Source: CAD feature listing. Evaluate the final solid. Frame: model axes, mm. A direction names the side the tool comes from. Give positions to 0.01 mm unless a question says otherwise; leave off trailing zeros. Order: outer loops, then holes, each group sorted by start corner. A loop starts at its lowest first (then second) coordinate and runs counter-clockwise, first axis right, second up.
from build123d import *

# Parameters (mm, degrees)
F0_R      = 3.91
F1_DEPTH  = 25
F1_FACE_R = 3.91
F2_DEPTH  = 2
F3_SIZE   = 1


with BuildPart() as f1:
    # F0 (on Top) → F1 (new body)
    with BuildSketch(Plane.XY):
        Circle(F0_R)
    extrude(amount=-F1_DEPTH)

    # F0 (on Top) + F1_face (on face) → F2 (join)
    with BuildSketch(Plane.XY):
        Polygon((5.284141717, -4.9639043418), (6.9409381205, 2.0942487932), (1.6567964035, 7.058153135), (-5.284141717, 4.9639043418), (-6.9409381205, -2.0942487932), (-1.6567964035, -7.058153135), align=None)
        Circle(F0_R, mode=Mode.SUBTRACT)
    with BuildSketch(Plane.XY):
        Circle(F1_FACE_R)
    extrude(amount=F2_DEPTH)

    # F3
    f3_edges = [f1.edges().sort_by_distance(p)[0] for p in [
        (-3.91, 0, -25),
    ]]
    chamfer(f3_edges, length=F3_SIZE)


solid = f1.part
1) Section query C-C on x = 0. Output: boundary loops of the cut face in (y, z), and give its area (3 significant figures).
Checks:
outline: (-6.56, 0) - (-3.91, 0) - (-3.91, -24) - (-2.91, -25) - (2.91, -25) - (3.91, -24) - (3.91, 0) - (6.56, 0) - (6.56, 2) - (-6.56, 2) - close
area: 221 mm2
2) Section query D-D on y = -4.25. Output: boundary loops of the cut face in (x, z).
Checks:
outline: (-4.65, 0) - (5.45, 0) - (5.45, 2) - (-4.65, 2) - close
3) Ray query, L1, parallel to Z at x = 1.75, y = -5.5; L2, parallel to Y at x = 0, z = -15.5; L3, parallel to Z at x = 3, y = 1.25. Return the intervals inside material, ascending.
Checks:
L1: z = 0 to 2
L2: y = -3.91 to 3.91
L3: z = -24.66 to 2
4) Reachability of faces 1 (the face through (-1.765, 6.026, 0.986)), 2 (the face through (3, -3, 0)) from +Z, -Z, +X, -X, +Y, -Y: full face, straight path, thin tool, end or side. Return the list, or none.
Checks:
face 1: +Z, -Z, -X, +Y
face 2: -Z
5) Section query A-A on z = -19.25. Output: boundary loops of the cut face in (x, y).
Checks:
outline: circle Ø7.82 at (0, 0)
6) First-contact query: pin 1 Ø2 at (y, z) = (-2.5, -3.5) entering from -X; pin 2 Ø1.5 at (x, z) = (-1.5, -1.5) entering from -Y; pin 3 Ø1 at (x, z) = (5.5, -13) entering from +Y; pin 4 Ø6 at (y, z) = (3, -21.5) entering from -X. Flat tips, straight axial feed; report the tip coordinate or a pass-through.
Checks:
pin 1: stops at x = -3.61
pin 2: stops at y = -3.84
pin 3: passes through
pin 4: stops at x = -3.91
7) Section query B-B on y = 0. Output: boundary loops of the cut face in (x, z), and give its area (3 significant figures).
Checks:
outline: (-6.45, 0) - (-3.91, 0) - (-3.91, -24) - (-2.91, -25) - (2.91, -25) - (3.91, -24) - (3.91, 0) - (6.45, 0) - (6.45, 2) - (-6.45, 2) - close
area: 220 mm2
